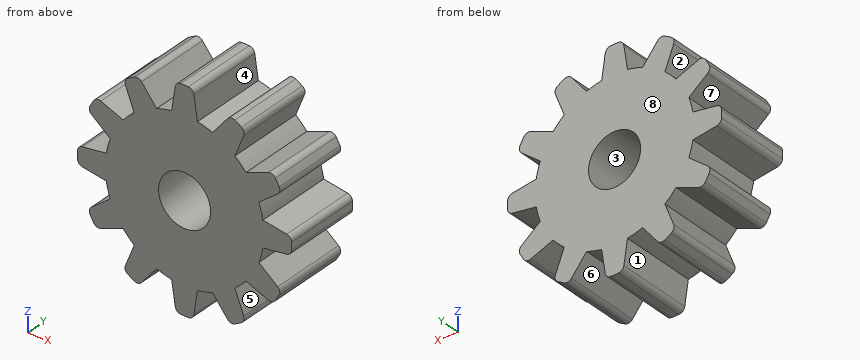
Autodesk Inventor part; units mm, degrees
ref_plane "YZ Plane" through (0, 0, 0) normal (1, 0, 0) x (0, 1, 0)
ref_plane "XZ Plane" through (0, 0, 0) normal (0, 1, 0) x (-1, 0, 0)
ref_plane "XY Plane" through (0, 0, 0) normal (0, 0, 1) x (1, 0, 0)
sketch "Sketch1" plane through (0, 0, 0) normal (0, 1, 0) x (-1, 0, 0)
  arc A0 (0.45, -5.5819) -> (-0.45, -5.5819) centre (0, 0) ccw construction
  circle A1 centre (0, 0) radius 4.15
  line L0 (-0.45, -5.5819) -> (-0.675, -4.0947)
  line L1 (0.675, -4.0947) -> (0.45, -5.5819)
  line L2 (0.675, -4.0947) -> (-0.675, -4.0947) construction
  line L3 (0.45, -5.5819) -> (-0.45, -5.5819) construction
  arc A2 (-0.45, -5.5819) -> (0.45, -5.5819) centre (0, 0) ccw
  circle A3 centre (0, 0) radius 1.3625
  dimension "d1" = 11.2
  dimension "d2" = 8.3
  dimension "d3" = 0.9
  dimension "d4" = 1.35
  dimension "d13" = 2.725
extrude "Extrusion1" add sketch "Sketch1" along normal blind 4 contours A1 | A3
extrude "Extrusion2" add sketch "Sketch1" along normal blind 4 contours A1 L1 A2 L0
fillet "Fillet1" radius 0.3 2 edges at (0.45, 2, -5.5819) (-0.45, 2, -5.5819)
pattern_circular "Circular Pattern1" count 12 over 360 about axis through (0, 0, 0) along (0, 1, 0) of "Extrusion2", "Fillet1"
extrude "Extrusion3" cut sketch "Sketch1" along normal blind 4 contours A3
properties part number "Motor Shaft Gear" material "ABS Plastic"
CAD build for the part. Positions are in the model's coordinates, mm. Face numbers are marked on the shaded views. A direction names the side the tool comes from. Round coordinates to 2 decimals unless told otherwise and drop trailing zeros. Write each loop counter-clockwise with the first axis right and the second up, starting at its lowest first coordinate (ties: lowest second). Pieces come first, ordered by that corner, then holes. Notation, with made-up numbers: (27, 89.25) - (70, 89.25) arc R19 cw to (70, 102.25) - close; hole circle Ø10 at (74.5, 23). An arc over 180 degrees is marked (long way). Return JSON: item names as keys, results as strings. Group by question number.
Item 1: Band-saw the part on D-D on z = -1.75. List the corners of the cut face in (x, y), plus the area to 3 significant figures.
Item 2: Probe probe 1 along Z at (x, y) = (0, 1.5); probe 2 along X at (y, z) = (0.5, 4.25); probe 3 along Z at (x, y) = (-4.75, 1.2). List the from-to ranges inside material, lowest first.
Item 3: Band-saw the part on C-C on x = 4.25. List the corners of the cut face in (y, z), plus the area to 3 significant figures.
Item 4: Band-saw the part on A-A on x = 0. List the corners of the cut face in (y, z), plus the area to 3 significant figures.
Item 5: Band-saw the part on B-B on z = 0. List the corners of the cut face in (x, y), plus the area to 3 significant figures.
Item 6: Mould opens along X. For the marked faces 6, 7 and 8 say: +X half, -X half, draft (parallel to the pull), parting line (faces both ways), or undercut.
Item 7: 3-axis set-ups, long thin cutter, end or side, ignore diameter. For the marked faces 1, 2, 3, 4 and 5: which of +Z, -Z, +X, -X, +Y, -Y reach the whole face in a straight line?
Item 8: Flat gauge pin, fed straight in: pin 1 Ø4 at (x, z) = (-4, 3) entering from +Y. Where does the tip first touch, or does it go through?
Resolved:
{
 "1": {"outline": "(-4.24, 0) - (4.24, 0) - (4.24, 4) - (-4.24, 4) - close", "area": "33.9 mm²"},
 "2": {"probe 1": "z = -5.6 to -1.36, 1.36 to 5.6", "probe 2": "x = -3.04 to -1.76, -0.65 to 0.65, 1.76 to 3.04", "probe 3": "z = -2.97 to -2.15, -0.58 to 0.58, 2.15 to 2.97"},
 "3": {"outline": "(0, -3.04) - (4, -3.04) - (4, -1.76) - (0, -1.76) - close; (0, -0.65) - (4, -0.65) - (4, 0.65) - (0, 0.65) - close; (0, 1.76) - (4, 1.76) - (4, 3.04) - (0, 3.04) - close", "area": "15.5 mm²"},
 "4": {"outline": "(0, -5.6) - (4, -5.6) - (4, -1.36) - (0, -1.36) - close; (0, 1.36) - (4, 1.36) - (4, 5.6) - (0, 5.6) - close", "area": "33.9 mm²"},
 "5": {"outline": "(-5.6, 0) - (-1.36, 0) - (-1.36, 4) - (-5.6, 4) - close; (1.36, 0) - (5.6, 0) - (5.6, 4) - (1.36, 4) - close", "area": "33.9 mm²"},
 "6": {"face 6": "undercut", "face 7": "-X half", "face 8": "draft"},
 "7": {"face 1": "-Z, +Y, -Y", "face 2": "-X, +Y, -Y", "face 3": "+Y, -Y", "face 4": "+Z, +Y, -Y", "face 5": "+X, +Y, -Y"},
 "8": {"pin 1": "stops at y = 4"}
}
